Input: dimensioned drawing with shaded views. Units: mm. Origin: part minimum x, y, z. A direction names the side the tool comes from. Coordinates: 2 decimals unless noted, no trailing zeros. Order: outer loops, then holes, each group sorted by start corner. A loop starts at its lowest first (then second) coordinate and runs counter-clockwise, first axis right, second up. Notation, with made-up numbers: (32, -11) - (39, -11) arc R24 cw to (39, 7) - close; hole circle Ø6 at (18.5, 4). An arc over 180 degrees is marked (long way). Answer as CSV lines item,"result". Start each with the question number.
Item 1: Section B-B (x = 56). Output: boundary loops of the cut face in (y, z), and give its area (3 significant figures).
Item 2: Draft query along Y for the marked faces 3, 4 and 5. Return one class per face: +Y half, -Y half, draft (parallel to the pull), parting line (faces both ways), or undercut.
Item 3: Section D-D (z = 10.75). Output: boundary loops of the cut face in (x, y), and give its area (3 significant figures).
Item 4: Material intervals for line 1 along Y through (x, z) = (46, 4.25); line 2 along Y through (x, z) = (38, 3.5); line 3 along Y through (x, z) = (14.5, 16.25), sorted ascending.
Item 5: First-contact query: pin 1 (1 mm diameter, centred on x = 30.5, y = 11.5, fed in from +Z). Flat tip, straight axial feed; report the tip coordinate or a pass-through.
Item 6: Section C-C (z = 2). Output: boundary loops of the cut face in (x, y), and give its area (3 significant figures).
Item 7: Access query for the marked faces 1 and 2. Directions: +Z, -Z, +X, -X, +Y, -Y. A direction counts if a zero-diameter tool reaches every point of the face in a straight line with its end or side. Return the directions, or none.
Item 8: Section A-A (y = 20). Output: boundary loops of the cut face in (x, z), and give its area (3 significant figures).
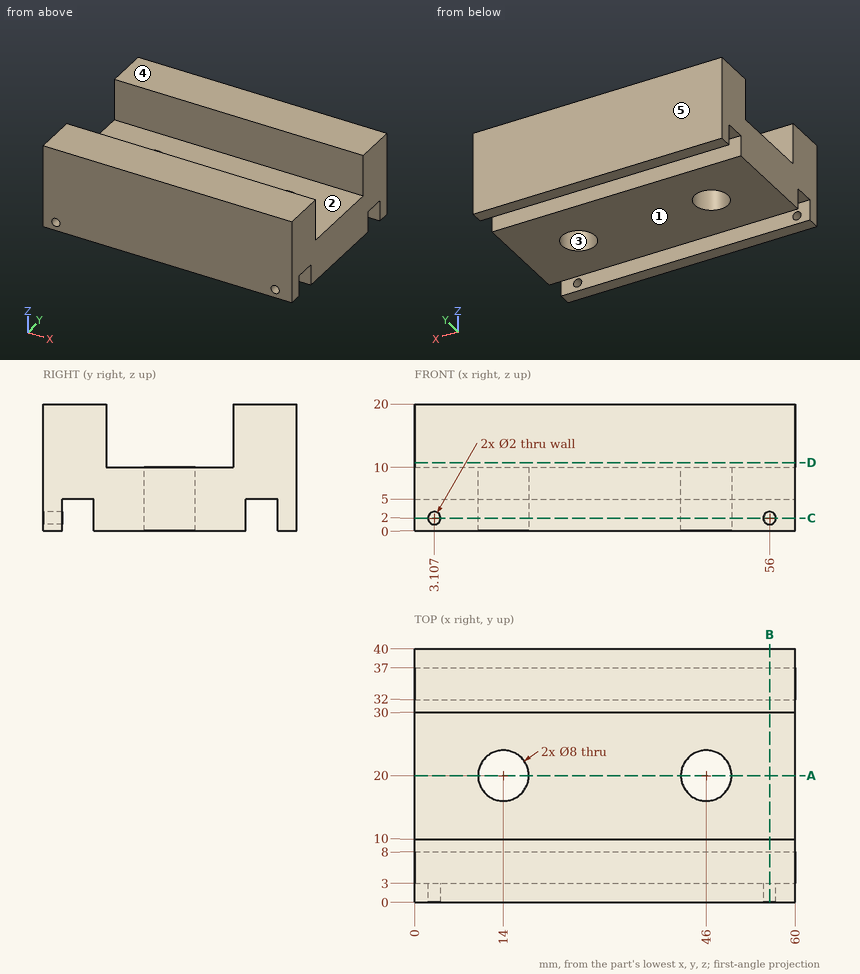
Determined:
1,outline,"(0, 0) - (3, 0) - (3, 1) - (0, 1) - close; (0, 3) - (3, 3) - (3, 5) - (8, 5) - (8, 0) - (32, 0) - (32, 5) - (37, 5) - (37, 0) - (40, 0) - (40, 20) - (30, 20) - (30, 10) - (10, 10) - (10, 20) - (0, 20) - close"
1,area,"544 mm^2"
2,face 3,"undercut"
2,face 4,"draft"
2,face 5,"+Y half"
3,outline,"(0, 0) - (60, 0) - (60, 10) - (0, 10) - close; (0, 30) - (60, 30) - (60, 40) - (0, 40) - close"
3,area,"1,200 mm^2"
4,line 1,"y = 0 to 3, 8 to 16, 24 to 32, 37 to 40"
4,line 2,"y = 0 to 3, 8 to 32, 37 to 40"
4,line 3,"y = 0 to 10, 30 to 40"
5,pin 1,"stops at z = 10"
6,outline,"(0, 0) - (2.11, 0) - (2.11, 3) - (0, 3) - close; (0, 8) - (60, 8) - (60, 32) - (0, 32) - close; (0, 37) - (60, 37) - (60, 40) - (0, 40) - close; (4.11, 0) - (55, 0) - (55, 3) - (4.11, 3) - close; (57, 0) - (60, 0) - (60, 3) - (57, 3) - close; hole circle Ø8 at (14, 20); hole circle Ø8 at (46, 20)"
6,area,"1,690 mm^2"
7,face 1,"-Z, +X, -X, +Y, -Y"
7,face 2,"+Z, +X, -X"
8,outline,"(0, 0) - (10, 0) - (10, 10) - (0, 10) - close; (18, 0) - (42, 0) - (42, 10) - (18, 10) - close; (50, 0) - (60, 0) - (60, 10) - (50, 10) - close"
8,area,"440 mm^2"
